Autodesk Inventor part; units mm, degrees
ref_plane "Work Plane1" through (0, 0, 70) normal (0, 0, 1) x (1, 0, 0)
ref_plane "YZ Plane" through (0, 0, 0) normal (1, 0, 0) x (0, 1, 0)
ref_plane "XZ Plane" through (0, 0, 0) normal (0, 1, 0) x (-1, 0, 0)
sketch "Sketch1" plane through (0, 0, 0) normal (0, 0, 1) x (1, 0, 0)
  line L0 (-25, -27.5) -> (25, -27.5)
  line L1 (25, -27.5) -> (25, 27.5)
  line L2 (25, 27.5) -> (-25, 27.5)
  line L3 (-25, 27.5) -> (-25, -27.5)
  line L4 (-25, -27.5) -> (25, 27.5) construction
  line L5 (25, -27.5) -> (-25, 27.5) construction
  point P0 (0, 0)
  dimension "d0" = 50
  dimension "d1" = 55
extrude "Extrusion1" add sketch "Sketch1" along normal blind 10
ref_plane "Work Plane1" through (0, 0, 70) normal (0, 0, 1) x (1, 0, 0)
sketch "Sketch3" plane through (0, 0, 70) normal (0, 0, 1) x (1, 0, 0)
  line L0 (-50, -50) -> (50, -50)
  line L1 (50, -50) -> (50, 50)
  line L2 (50, 50) -> (-50, 50)
  line L3 (-50, 50) -> (-50, -50)
  line L4 (-50, -50) -> (50, 50) construction
  line L5 (50, -50) -> (-50, 50) construction
  line L6 (-42.5, -42.5) -> (42.5, 42.5) construction
  line L7 (42.5, -42.5) -> (-42.5, 42.5) construction
  point P0 (0, 0)
  dimension "d9" = 100
  dimension "d10" = 100
extrude "Extrusion3" add sketch "Sketch3" along normal blind 5
loft "Loft1" add section 1 edges at (0, -27.5, 10) (25, 0, 10) (0, 27.5, 10) (-25, 0, 10) section 2 edges at (0, -50, 70) (-50, 0, 70) (0, 50, 70) (50, 0, 70)
shell "Shell2" thickness 5 removed faces 1 at (-16.6667, 16.6667, 75)
sketch "Sketch4" plane through (25, -27.5, 0) normal (1, 0, 0) x (0, 0, -1)
  line L0 (0, 55) -> (-10, 55)
  line L1 (0, 0) -> (-10, 0)
  line L2 (-3, 55) -> (-7, 55)
  line L3 (-7, 55) -> (-7, 5)
  line L4 (-7, 5) -> (-3, 5)
  line L5 (-3, 5) -> (-3, 55)
  point P0 (0, 27.5)
  dimension "d28" = 4
  dimension "d29" = 3
  dimension "d30" = 5
extrude "Extrusion4" cut sketch "Sketch4" against normal up to surface (45 mm away)
sketch "Sketch5" plane through (0, 0, 0) normal (0, 0, -1) x (-1, 0, 0)
  line L0 (-20, 22.5) -> (20, 22.5) construction
  line L1 (20, 22.5) -> (-20, 22.5)
  line L2 (20, -22.5) -> (20, 52.5) construction
  arc A0 (-20, -10.9429) -> (20, -22.5) centre (20, 52.5) ccw
  line L3 (20, -22.5) -> (20, 22.5)
  line L4 (-20, 22.5) -> (-20, -22.5)
  line L5 (-20, 22.5) -> (-20, -22.5)
  line L6 (-20, -22.5) -> (-20, -22.535)
  line L7 (-20, -22.535) -> (-20, 22.535)
  line L8 (-20, 22.5) -> (-20, 22.535)
  line L9 (-20, -10.9429) -> (-20, 22.5)
  line L10 (20, 22.5) -> (-20, 22.5)
  point P0 (0, 0)
  dimension "d31" = 75
extrude "Extrusion5" cut sketch "Sketch5" against normal through all
properties part number "funnel_"
For this review, take the finished solid that the model builds, in its own axes (mm). A direction names the side the tool comes from. Coordinates: 2 decimals unless noted, no trailing zeros.
(1) The part is to be moulded in two halves that separate along X. For faces 1 (the face through (-25, 0, 5)), 2 (the face through (11, -18, 0)), 3 (the face through (25, -0.4, 2.7)), 4 (the face through (0, 22.5, 9)), say which applies: +X half, -X half, draft (parallel to the pull), parting line (faces both ways), or undercut.
(2) Tool access review of faces 5 (the face through (0, -27.5, 5)), 6 (the face through (0, 22.5, 1)), 7 (the face through (20, 0, 9)), 8 (the face through (0.3, 27.5, 2.7)), 9 (the face through (21, 6, 3)): name each direction out of +Z, -Z, +X, -X, +Y, -Y from which nothing blocks a thin tool from reaching the whole face with its end or side.
(3) For pin 1 Ø8.5 at (x, z) = (12.5, 5.5) entering from +Y; pin 2 Ø4.5 at (y, z) = (-7.5, 8.5) entering from -X; pin 3 Ø3.5 at (y, z) = (8, 2) entering from -X; pin 4 Ø13.5 at (x, y) = (7, 0.5) entering from -Z, all flat-tipped, find the tip position at first contact; note any pin that passes through.
(4) Add section A-A on x = 10. Count the separate pieces of the cut face and the enclosed holes in it, then the cut area to 3 significant figures.
(5) Wall thickness on probe 1 along X at (y, z) = (-20, 72.5); probe 2 along X at (y, z) = (-19, 37); probe 3 along Z at (x, y) = (23.5, 20.5): over which ranges is each line inside the solid? List them lowest first.
Answer sheet:
1. face 1: -X half
1. face 2: draft
1. face 3: +X half
1. face 4: undercut
2. face 5: -Z, +X, -X, -Y
2. face 6: +Z, -Z
2. face 7: +Z
2. face 8: -Z, +X, -X, +Y
2. face 9: +X, +Y
3. pin 1: stops at y = 27.5
3. pin 2: stops at x = -25.31
3. pin 3: stops at x = -25
3. pin 4: passes through
4. separate pieces: 3
4. enclosed holes: 0
4. area: 790 mm2
5. probe 1: x = -50 to -45, 45 to 50
5. probe 2: x = -36.25 to -30.83, 30.83 to 36.25
5. probe 3: z = 0 to 3, 7 to 19.4
